Geometry: see drawing. Coordinates: mm, zero at the bounding-box minimum. A direction names the side the tool comes from. Round coordinates to 2 decimals unless told otherwise and drop trailing zeros. Loops run counter-clockwise (first coordinate to the right, second up) from the corner with the lowest first, then second, coordinate; pieces in that order, holes last. Notation, with made-up numbers: (86.5, 45) - (138.5, 45) arc R15 cw to (138.5, 50) - close; hole circle Ø10 at (39.5, 7). An arc over 180 degrees is marked (long way). Use CSV: the item, a comma, the result in double quotes. Start each with the question number.
1. Access query for the marked faces 1, 2 and 3. Directions: +Z, -Z, +X, -X, +Y, -Y. A direction counts if a zero-diameter tool reaches every point of the face in a straight line with its end or side. Return the directions, or none.
2. Pin query (flat end, axial travel): P1, Ø12, axis at y = 38, z = 37.5, coming from the +X side; P2, Ø5, axis at y = 18.5, z = 69.5, coming from the -X side; P3, Ø4.5, axis at x = 96, y = 29.5, coming from the +Z side; P4, Ø12, axis at x = 89, z = 6.5, coming from the +Y side. Return the tip coordinate at first contact, or that it passes through.
3. Cut plane D-D (z = 44). Return loops of the section in (x, y).
4. Cut plane C-C (y = 49). Return loops of the section in (x, z).
5. Pull-direction query (X, two-part tool) for the marked faces 4, 5 and 6; classes: +X half, -X half, draft (parallel to the pull), parting line (faces both ways), or undercut.
6. Cut plane A-A (x = 95). Return loops of the section in (y, z).
7. Material intervals for probe 1 along Z at (x, y) = (95, 27); probe 2 along X at (y, z) = (28.25, 6); probe 3 along X at (y, z) = (19.5, 14), sorted ascending. Write a range as from..to.
8. Cut plane B-B (z = 6). Return loops of the section in (x, y).
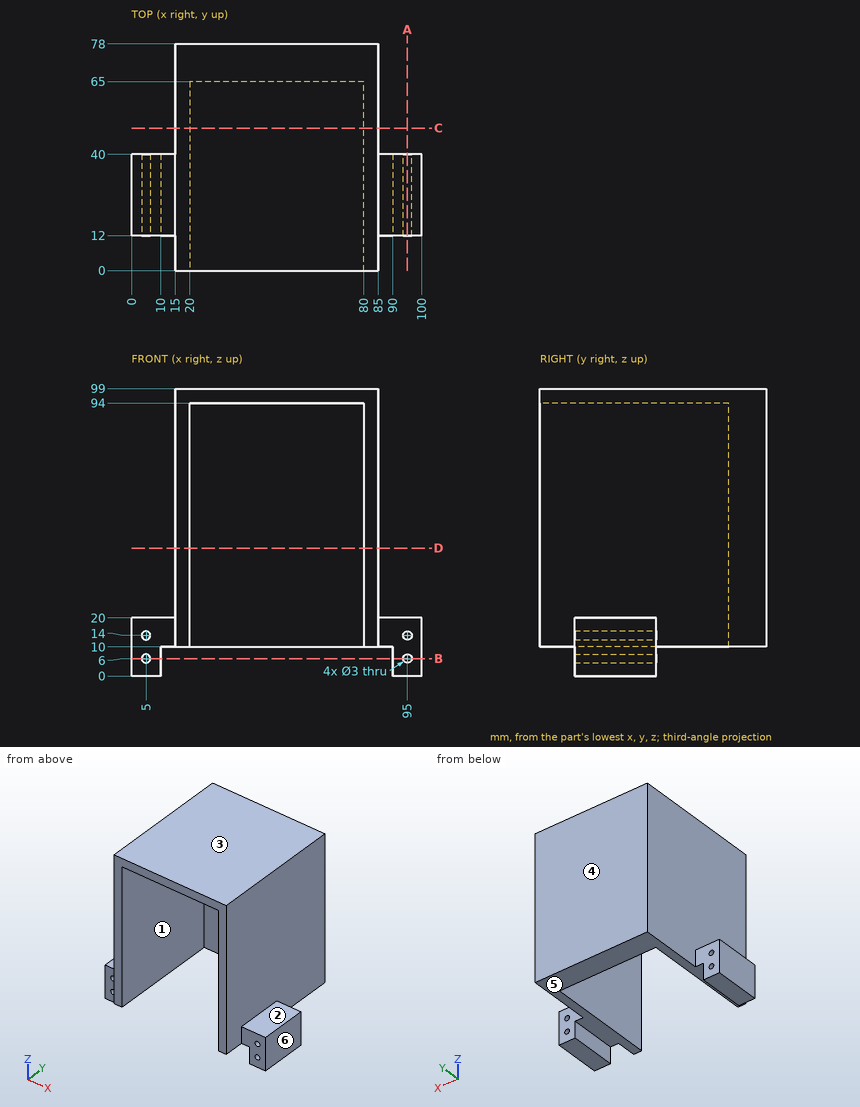
Established:
1,face 1,"-Z, -Y"
1,face 2,"+Z, +X, +Y, -Y"
1,face 3,"+Z, +X, -X, +Y, -Y"
2,P1,"stops at x = 85"
2,P2,"stops at x = 15"
2,P3,"stops at z = 20"
2,P4,"stops at y = 78"
3,outline,"(15, 0) - (20, 0) - (20, 65) - (80, 65) - (80, 0) - (85, 0) - (85, 78) - (15, 78) - close"
4,outline,"(15, 10) - (20, 10) - (20, 94) - (80, 94) - (80, 10) - (85, 10) - (85, 99) - (15, 99) - close"
5,face 4,"draft"
5,face 5,"undercut"
5,face 6,"+X half"
6,outline,"(12, 0) - (40, 0) - (40, 4.5) - (12, 4.5) - close; (12, 7.5) - (40, 7.5) - (40, 12.5) - (12, 12.5) - close; (12, 15.5) - (40, 15.5) - (40, 20) - (12, 20) - close"
7,probe 1,"z = 0..4.5, 7.5..12.5, 15.5..20"
7,probe 2,"x = 0..3.5, 6.5..10, 90..93.5, 96.5..100"
7,probe 3,"x = 0..3.5, 6.5..20, 80..93.5, 96.5..100"
8,outline,"(0, 12) - (3.5, 12) - (3.5, 40) - (0, 40) - close; (6.5, 12) - (10, 12) - (10, 40) - (6.5, 40) - close; (90, 12) - (93.5, 12) - (93.5, 40) - (90, 40) - close; (96.5, 12) - (100, 12) - (100, 40) - (96.5, 40) - close"
